Geometry: final body of the model. Coordinates: model frame, mm. A direction names the side the tool comes from. Round coordinates to 2 decimals unless told otherwise and drop trailing zeros. Write each loop counter-clockwise with the first axis right and the second up, starting at its lowest first coordinate (ties: lowest second). Pieces come first, ordered by that corner, then holes.
from build123d import *

# Parameters (mm, degrees)
SKETCH1_W           = 25
SKETCH1_H           = 52
BOSS_EXTRUDE1_DEPTH = 7
SKETCH2_R           = 0.9
CUT_EXTRUDE1_DEPTH  = 30.685855218
LPATTERN1_COUNT     = 6
LPATTERN1_PITCH     = 8
SKETCH5_R           = 4
BOSS_EXTRUDE2_DEPTH = 22
SKETCH6_R           = 5
SKETCH6_R_2         = 4
BOSS_EXTRUDE3_DEPTH = 5
CUT_EXTRUDE2_START  = -10
CUT_EXTRUDE2_DEPTH  = 10
SKETCH9_R           = 1.875
CUT_EXTRUDE3_DEPTH  = 3.5
LPATTERN2_COUNT     = 6
LPATTERN2_PITCH     = 8
CHAMFER2_SIZE       = 3
CHAMFER2_SIZE_2     = 5
SKETCH10_W          = 14.9
SKETCH10_H          = 52
CUT_EXTRUDE4_DEPTH  = 2
CHAMFER3_SIZE       = 2


# Some blends are built 0.0001 mm under size
with BuildPart() as part:
    # Sketch1 → Boss-Extrude1 (new body)
    with BuildSketch(Plane(origin=(0, 0, 0), x_dir=(1, 0, 0), z_dir=(0, 1, 0))):
        Rectangle(SKETCH1_W, SKETCH1_H)
    extrude(amount=BOSS_EXTRUDE1_DEPTH)

    # Sketch2 → Cut-Extrude1 (cut, through all)
    with BuildSketch(Plane(origin=(0, 7, 0), x_dir=(1, 0, 0), z_dir=(0, 1, 0))):
        with Locations(Location((-10.45, -20, 0), (0, 0, 270))):
            Circle(SKETCH2_R)
        with Locations(Location((10.45, -20, 0), (0, 0, 270))):
            Circle(SKETCH2_R)
    cut_extrude1 = extrude(amount=-CUT_EXTRUDE1_DEPTH, mode=Mode.SUBTRACT)

    # LPattern1: Cut-Extrude1 ×6
    with Locations(*[(0, 0, -i * LPATTERN1_PITCH) for i in range(1, LPATTERN1_COUNT)]):
        add(cut_extrude1, mode=Mode.SUBTRACT)

    # Sketch5 → Boss-Extrude2 (add)
    with BuildSketch(Plane(origin=(0, 7, 0), x_dir=(1, 0, 0), z_dir=(0, 1, 0))):
        with Locations(Location((0, 0, 0), (0, 0, 90))):
            Circle(SKETCH5_R)
    extrude(amount=BOSS_EXTRUDE2_DEPTH)

    # Sketch6 → Boss-Extrude3 (add)
    with BuildSketch(Plane(origin=(0, 7, 0), x_dir=(1, 0, 0), z_dir=(0, 1, 0))):
        with Locations(Location((0, 0, 0), (0, 0, 90))):
            Circle(SKETCH6_R)
        with Locations(Location((0, 0, 0), (0, 0, 270))):
            Circle(SKETCH6_R_2, mode=Mode.SUBTRACT)
    extrude(amount=BOSS_EXTRUDE3_DEPTH)

    # Sketch8 → Cut-Extrude2 (cut)
    with BuildSketch(Plane(origin=(0, 29, 0), x_dir=(1, 0, 0), z_dir=(0, 1, 0)).offset(CUT_EXTRUDE2_START)):
        with BuildLine():
            Line((-3.122498999, -2.5), (3.122498999, -2.5))
            ThreePointArc((3.122498999, -2.5), (0, -4), (-3.122498999, -2.5))
        make_face()
    extrude(amount=CUT_EXTRUDE2_DEPTH, mode=Mode.SUBTRACT)

    # Sketch9 → Cut-Extrude3 (cut)
    with BuildSketch(Plane(origin=(0, 7, 0), x_dir=(1, 0, 0), z_dir=(0, 1, 0))):
        with Locations(Location((-10.45, 20, 0), (0, 0, 270))):
            Circle(SKETCH9_R)
        with Locations(Location((10.45, 20, 0), (0, 0, 270))):
            Circle(SKETCH9_R)
    cut_extrude3 = extrude(amount=-CUT_EXTRUDE3_DEPTH, mode=Mode.SUBTRACT)

    # LPattern2: Cut-Extrude3 ×6
    with Locations(*[(0, 0, i * LPATTERN2_PITCH) for i in range(1, LPATTERN2_COUNT)]):
        add(cut_extrude3, mode=Mode.SUBTRACT)

    # Chamfer2
    # the kernel refuses this chamfer: 5, 3 mm, written as the material it takes off along each edge
    with BuildSketch(Plane(origin=(-12.5, 7, -38.931305486), x_dir=(-0.0551862070597658, -0.9984760801092616, 0), z_dir=(0, 0, 1)), Plane(origin=(12.5, 7, 38.931305486), x_dir=(0.0551862070597658, -0.9984760801092616, 0), z_dir=(0, 0, -1))) as chamfer2_piece_1:
        Polygon((CHAMFER2_SIZE * 0.998476080109, CHAMFER2_SIZE * 0.0551862070598), (-CHAMFER2_SIZE_2 * 0.0551862070598, CHAMFER2_SIZE_2 * 0.998476080109), (0, 0), align=None)
    extrude(amount=77.862610972, mode=Mode.SUBTRACT)

    # Sketch10 → Cut-Extrude4 (cut)
    with BuildSketch(Plane.XZ):
        Rectangle(SKETCH10_W, SKETCH10_H)
    extrude(amount=-CUT_EXTRUDE4_DEPTH, mode=Mode.SUBTRACT)

    # Chamfer3
    chamfer3_edges = [part.edges().sort_by_distance(p)[0] for p in [
        (7.45, 2, 0),
        (-7.45, 2, 0),
    ]]
    chamfer(chamfer3_edges, length=CHAMFER3_SIZE - 0.0001)  # a hair under: the kernel refuses the full size


solid = part.part
1) Section A-A on x = 0. Output: boundary loops of the cut face in (y, z), plus the area to 3 significant figures.
2) First-contact query: P1, Ø1.9, axis at x = 10, z = 3, coming from the +Y side; P2, Ø1.1, axis at x = 10.5, z = 19.5, coming from the +Y side; P3, Ø1.5, axis at x = -10, z = -2, coming from the +Y side. Flat tips, straight axial feed; report the tip coordinate or a pass-through.
3) Reachability of faces 4 (the flat face through (-10, 3.5, -3)), 5 (the cylindrical face through (-11.329, 1.774, 3.805)), 6 (the flat face through (0, 19, 3)), 7 (the flat face through (-6.44, 1.01, -0.36)) from +Z, -Z, +X, -X, +Y, -Y: full face, straight path, thin tool, end or side. Return the list, or none.
4) Line query: probe 1 along X at (y, z) = (1.75, 12); probe 2 along X at (y, z) = (1.5, 4); probe 3 along X at (y, z) = (5, -12) (3 decimals). Output: solid intervals per line, ascending.
5) Draft query along Z for faces 1 (the flat face through (10, 0, 0)), 2 (the flat face through (11, 3.5, 5)), 3 (the flat face through (0, 3, 26)). Return one class per face: pulls with the +Z half, pulls with the -Z half, needs draft (parallel to the pull), parting line crosses it, or undercut.
6) Section B-B on z = -20. State how many separate pieces and enclosed holes the cut face has, plus the area to 3 significant figures.
Filled in:
1. outline: (2, -26) - (7, -26) - (7, -5) - (12, -5) - (12, -4) - (29, -4) - (29, 2.5) - (19, 2.5) - (19, 4) - (12, 4) - (12, 5) - (7, 5) - (7, 26) - (2, 26) - close
1. area: 431 mm2
2. P1: stops at y = 6.04
2. P2: stops at y = 3.5
2. P3: stops at y = 5.95
3. face 4: +Y
3. face 5: +Y, -Y
3. face 6: +Z, +X, -X, +Y
3. face 7: +Z, -Z, -Y
4. probe 1: x = -12.5 to -11.35, -9.55 to -5.7, 5.7 to 9.55, 11.35 to 12.5
4. probe 2: x = -12.5 to -11.35, -9.55 to -5.95, 5.95 to 9.55, 11.35 to 12.5
4. probe 3: x = -8.575 to 8.575
5. face 1: needs draft
5. face 2: undercut
5. face 3: pulls with the +Z half
6. separate pieces: 3
6. enclosed holes: 0
6. area: 109 mm2
